Here's how the part is built. I have some questions about the finished solid (model axes, mm). Face numbers are marked on the shaded views. A direction names the side the tool comes from. Round coordinates to 2 decimals unless told otherwise and drop trailing zeros. Order: outer loops, then holes, each group sorted by start corner. A loop starts at its lowest first (then second) coordinate and runs counter-clockwise, first axis right, second up. Notation, with made-up numbers: M 5,14 L 53,14 A6 ccw 53,21 Z; hole C 22,-31 d3. An arc over 180 degrees is marked long. Use one line per item in the form item = value. Start each with the question number.
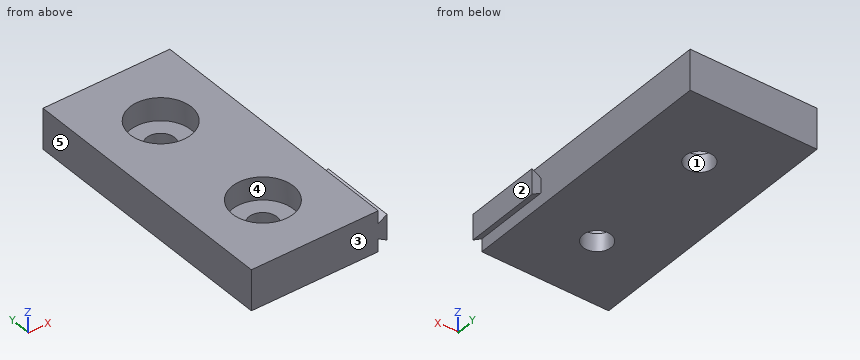
```python
from build123d import *

# Parameters (mm, degrees)
SKETCH2_W           = 25
SKETCH2_H           = 53
SKETCH2_R           = 2.75
BOSS_EXTRUDE1_DEPTH = 8
BOSS_EXTRUDE2_DEPTH = 15
SKETCH4_R           = 6
CUT_EXTRUDE1_DEPTH  = 4.5


with BuildPart() as part:
    # Sketch2 → Boss-Extrude1 (new body)
    with BuildSketch(Plane.XY):
        with Locations((12.5, 26.5)):
            Rectangle(SKETCH2_W, SKETCH2_H)
        with Locations((12.5, 39.2)):
            Circle(SKETCH2_R, mode=Mode.SUBTRACT)
        with Locations((12.5, 13.2)):
            Circle(SKETCH2_R, mode=Mode.SUBTRACT)
    extrude(amount=BOSS_EXTRUDE1_DEPTH)

    # Sketch3 → Boss-Extrude2 (add)
    with BuildSketch(Plane.XZ):
        Polygon((25, 2.5), (26.732050808, 1.5), (26.732050808, 6.5), (25, 5.5), align=None)
    extrude(amount=-BOSS_EXTRUDE2_DEPTH)

    # Sketch4 → Cut-Extrude1 (cut)
    with BuildSketch(Plane.XY.offset(8)):
        with Locations((12.5, 39.2)):
            Circle(SKETCH4_R)
        with Locations((12.5, 13.2)):
            Circle(SKETCH4_R)
    extrude(amount=-CUT_EXTRUDE1_DEPTH, mode=Mode.SUBTRACT)


solid = part.part
```
1) If we section it at D-D on y = 13.2: Write out the boundary of the cut face in (x, z).
2) If we section it at A-A on y = 39.2: Write out the boundary of the cut face in (x, z).
3) If we mould it in two halves opening along Y, with no side actions, what happens to the marked faces 1, 2 and 3? For each: +Y half, -Y half, draft (parallel to the pull), parting line (faces both ways), or undercut.
4) Will these pins go through, and if not, where does the flat tip stop? pin 1 Ø9.5 at (x, y) = (12.5, 13.5) entering from +Z; pin 2 Ø0.5 at (x, z) = (26, 4.5) entering from +Y; pin 3 Ø4.5 at (x, y) = (12.5, 39.2) entering from +Z.
5) On a 3-axis mill with a long thin cutter (end or side, diameter ignored), from which of +Z, -Z, +X, -X, +Y, -Y can I reach the whole of each face in a straight line? I mean the marked faces 4 and 5. Say none if no direction works.
6) If I drill on line 1 (Y direction, x = 12.5, z = 1.8); line 2 (X direction, y = 39.2, z = 2.7); line 3 (Y direction, x = 7.5, z = 7.5), over which ranges is the centre line in solid material (lowest first)?
7) If we section it at B-B on x = 12.5: Write out the boundary of the cut face in (y, z), then the cut area to 4 significant figures.
8) If we section it at C-C on z = 4: Write out the boundary of the cut face in (x, y), then the cut area to 3 significant figures.
Completed:
q1.outline = M 0,0 L 9.75,0 L 9.75,3.5 L 6.5,3.5 L 6.5,8 L 0,8 Z; M 15.25,0 L 25,0 L 25,2.5 L 26.73,1.5 L 26.73,6.5 L 25,5.5 L 25,8 L 18.5,8 L 18.5,3.5 L 15.25,3.5 Z
q2.outline = M 0,0 L 9.75,0 L 9.75,3.5 L 6.5,3.5 L 6.5,8 L 0,8 Z; M 15.25,0 L 25,0 L 25,8 L 18.5,8 L 18.5,3.5 L 15.25,3.5 Z
q3.face_1 = undercut
q3.face_2 = draft
q3.face_3 = -Y half
q4.pin_1 = 3.5
q4.pin_2 = 15
q4.pin_3 = through
q5.face_4 = +Z
q5.face_5 = +Z, -Z, -X, +Y, -Y
q6.line_1 = 0 to 10.45, 15.95 to 36.45, 41.95 to 53
q6.line_2 = 0 to 9.75, 15.25 to 25
q6.line_3 = 0 to 9.88, 16.52 to 35.88, 42.52 to 53
q7.outline = M 0,0 L 10.45,0 L 10.45,3.5 L 7.2,3.5 L 7.2,8 L 0,8 Z; M 15.95,0 L 36.45,0 L 36.45,3.5 L 33.2,3.5 L 33.2,8 L 19.2,8 L 19.2,3.5 L 15.95,3.5 Z; M 41.95,0 L 53,0 L 53,8 L 45.2,8 L 45.2,3.5 L 41.95,3.5 Z
q7.area = 277.5 mm²
q8.outline = M 0,0 L 26.73,0 L 26.73,15 L 25,15 L 25,53 L 0,53 Z; hole C 12.5,13.2 d12; hole C 12.5,39.2 d12
q8.area = 1,120 mm²
